Check sheet for the modelled part. Datum: model origin and axes. Units: mm. Face numbers are marked on the shaded views. A direction names the side the tool comes from. Give positions to 0.01 mm unless a question says otherwise; leave off trailing zeros. Order: outer loops, then holes, each group sorted by start corner. A loop starts at its lowest first (then second) coordinate and runs counter-clockwise, first axis right, second up.
```python
from build123d import *

# Parameters (mm, degrees)
SKETCH1_R                    = 27.125
BOSS_EXTRUDE1_DEPTH          = 6
CUT_EXTRUDE1_START           = 6
SKETCH2_R                    = 2.6
CUT_EXTRUDE1_DEPTH           = 45.826939745
CUT_EXTRUDE1_DRAFT           = 2
CUT_EXTRUDE1_PROFILE_2_DEPTH = 45.826939745
CUT_EXTRUDE1_PROFILE_2_DRAFT = 2
CUT_EXTRUDE1_PROFILE_3_DEPTH = 45.826939745
CUT_EXTRUDE1_PROFILE_3_DRAFT = 2
SKETCH2_R_2                  = 2.1
CUT_EXTRUDE1_PROFILE_4_DEPTH = 45.826939745
CUT_EXTRUDE1_PROFILE_4_DRAFT = 2
CUT_EXTRUDE1_PROFILE_5_DEPTH = 45.826939745
CUT_EXTRUDE1_PROFILE_5_DRAFT = 2
CUT_EXTRUDE1_PROFILE_6_DEPTH = 45.826939745
CUT_EXTRUDE1_PROFILE_6_DRAFT = 2
CUT_EXTRUDE1_PROFILE_7_DEPTH = 45.826939745
CUT_EXTRUDE1_PROFILE_7_DRAFT = 2
CUT_EXTRUDE1_PROFILE_8_DEPTH = 45.826939745
CUT_EXTRUDE1_PROFILE_8_DRAFT = 2
CUT_EXTRUDE1_PROFILE_9_DEPTH = 45.826939745
CUT_EXTRUDE1_PROFILE_9_DRAFT = 2


with BuildPart() as part:
    # Sketch1 → Boss-Extrude1 (new body)
    with BuildSketch(Plane(origin=(0, 0, 0), x_dir=(0, 1, 0), z_dir=(0, 0, 1))):
        with Locations(Location((0, 0, 0), (0, 0, 270))):
            Circle(SKETCH1_R)
    extrude(amount=BOSS_EXTRUDE1_DEPTH)


with BuildPart() as cut_extrude1_tool:
    # Sketch2 → Cut-Extrude1 (with draft: the straight prism first)
    with BuildSketch(Plane(origin=(0, 0, 6), x_dir=(1, 0, 0), z_dir=(0, 0, -1)).offset(CUT_EXTRUDE1_START)):
        with Locations((0, 16)):
            Circle(SKETCH2_R)
    extrude(amount=-CUT_EXTRUDE1_DEPTH)
    # Cut-Extrude1: the draft: its side faces are tilted about the plane it starts from
    cut_extrude1_sides = [cut_extrude1_tool.faces().sort_by_distance(p)[0] for p in [
        (-2.6, -16, 22.913469873),
    ]]
    draft(cut_extrude1_sides, Plane(origin=(0, 0, 6), x_dir=(1, 0, 0), z_dir=(0, 0, -1)).offset(CUT_EXTRUDE1_START), CUT_EXTRUDE1_DRAFT)


with BuildPart() as part_1:
    add(part.part)

    # Cut-Extrude1: cut by cut_extrude1_tool
    add(cut_extrude1_tool.part, mode=Mode.SUBTRACT)


with BuildPart() as cut_extrude1_profile_2_tool:
    # Sketch2 → Cut-Extrude1 profile 2 (with draft: the straight prism first)
    with BuildSketch(Plane(origin=(0, 0, 6), x_dir=(1, 0, 0), z_dir=(0, 0, -1)).offset(CUT_EXTRUDE1_START)):
        with Locations((13.856406461, -8)):
            Circle(SKETCH2_R)
    extrude(amount=-CUT_EXTRUDE1_PROFILE_2_DEPTH)
    # Cut-Extrude1 profile 2: the draft: its side faces are tilted about the plane it starts from
    cut_extrude1_profile_2_sides = [cut_extrude1_profile_2_tool.faces().sort_by_distance(p)[0] for p in [
        (11.256406461, 8, 22.913469873),
    ]]
    draft(cut_extrude1_profile_2_sides, Plane(origin=(0, 0, 6), x_dir=(1, 0, 0), z_dir=(0, 0, -1)).offset(CUT_EXTRUDE1_START), CUT_EXTRUDE1_PROFILE_2_DRAFT)


with BuildPart() as part_2:
    add(part_1.part)

    # Cut-Extrude1 profile 2: cut by cut_extrude1_profile_2_tool
    add(cut_extrude1_profile_2_tool.part, mode=Mode.SUBTRACT)


with BuildPart() as cut_extrude1_profile_3_tool:
    # Sketch2 → Cut-Extrude1 profile 3 (with draft: the straight prism first)
    with BuildSketch(Plane(origin=(0, 0, 6), x_dir=(1, 0, 0), z_dir=(0, 0, -1)).offset(CUT_EXTRUDE1_START)):
        with Locations((-13.856406461, -8)):
            Circle(SKETCH2_R)
    extrude(amount=-CUT_EXTRUDE1_PROFILE_3_DEPTH)
    # Cut-Extrude1 profile 3: the draft: its side faces are tilted about the plane it starts from
    cut_extrude1_profile_3_sides = [cut_extrude1_profile_3_tool.faces().sort_by_distance(p)[0] for p in [
        (-16.456406461, 8, 22.913469873),
    ]]
    draft(cut_extrude1_profile_3_sides, Plane(origin=(0, 0, 6), x_dir=(1, 0, 0), z_dir=(0, 0, -1)).offset(CUT_EXTRUDE1_START), CUT_EXTRUDE1_PROFILE_3_DRAFT)


with BuildPart() as part_3:
    add(part_2.part)

    # Cut-Extrude1 profile 3: cut by cut_extrude1_profile_3_tool
    add(cut_extrude1_profile_3_tool.part, mode=Mode.SUBTRACT)


with BuildPart() as cut_extrude1_profile_4_tool:
    # Sketch2 → Cut-Extrude1 profile 4 (with draft: the straight prism first)
    with BuildSketch(Plane(origin=(0, 0, 6), x_dir=(1, 0, 0), z_dir=(0, 0, -1)).offset(CUT_EXTRUDE1_START)):
        with Locations((-9, -15.588457268)):
            Circle(SKETCH2_R_2)
    extrude(amount=-CUT_EXTRUDE1_PROFILE_4_DEPTH)
    # Cut-Extrude1 profile 4: the draft: its side faces are tilted about the plane it starts from
    cut_extrude1_profile_4_sides = [cut_extrude1_profile_4_tool.faces().sort_by_distance(p)[0] for p in [
        (-11.1, 15.588457268, 22.913469873),
    ]]
    draft(cut_extrude1_profile_4_sides, Plane(origin=(0, 0, 6), x_dir=(1, 0, 0), z_dir=(0, 0, -1)).offset(CUT_EXTRUDE1_START), CUT_EXTRUDE1_PROFILE_4_DRAFT)


with BuildPart() as part_4:
    add(part_3.part)

    # Cut-Extrude1 profile 4: cut by cut_extrude1_profile_4_tool
    add(cut_extrude1_profile_4_tool.part, mode=Mode.SUBTRACT)


with BuildPart() as cut_extrude1_profile_5_tool:
    # Sketch2 → Cut-Extrude1 profile 5 (with draft: the straight prism first)
    with BuildSketch(Plane(origin=(0, 0, 6), x_dir=(1, 0, 0), z_dir=(0, 0, -1)).offset(CUT_EXTRUDE1_START)):
        with Locations((-18, 0)):
            Circle(SKETCH2_R_2)
    extrude(amount=-CUT_EXTRUDE1_PROFILE_5_DEPTH)
    # Cut-Extrude1 profile 5: the draft: its side faces are tilted about the plane it starts from
    cut_extrude1_profile_5_sides = [cut_extrude1_profile_5_tool.faces().sort_by_distance(p)[0] for p in [
        (-20.1, 0, 22.913469873),
    ]]
    draft(cut_extrude1_profile_5_sides, Plane(origin=(0, 0, 6), x_dir=(1, 0, 0), z_dir=(0, 0, -1)).offset(CUT_EXTRUDE1_START), CUT_EXTRUDE1_PROFILE_5_DRAFT)


with BuildPart() as part_5:
    add(part_4.part)

    # Cut-Extrude1 profile 5: cut by cut_extrude1_profile_5_tool
    add(cut_extrude1_profile_5_tool.part, mode=Mode.SUBTRACT)


with BuildPart() as cut_extrude1_profile_6_tool:
    # Sketch2 → Cut-Extrude1 profile 6 (with draft: the straight prism first)
    with BuildSketch(Plane(origin=(0, 0, 6), x_dir=(1, 0, 0), z_dir=(0, 0, -1)).offset(CUT_EXTRUDE1_START)):
        with Locations((-9, 15.588457268)):
            Circle(SKETCH2_R_2)
    extrude(amount=-CUT_EXTRUDE1_PROFILE_6_DEPTH)
    # Cut-Extrude1 profile 6: the draft: its side faces are tilted about the plane it starts from
    cut_extrude1_profile_6_sides = [cut_extrude1_profile_6_tool.faces().sort_by_distance(p)[0] for p in [
        (-11.1, -15.588457268, 22.913469873),
    ]]
    draft(cut_extrude1_profile_6_sides, Plane(origin=(0, 0, 6), x_dir=(1, 0, 0), z_dir=(0, 0, -1)).offset(CUT_EXTRUDE1_START), CUT_EXTRUDE1_PROFILE_6_DRAFT)


with BuildPart() as part_6:
    add(part_5.part)

    # Cut-Extrude1 profile 6: cut by cut_extrude1_profile_6_tool
    add(cut_extrude1_profile_6_tool.part, mode=Mode.SUBTRACT)


with BuildPart() as cut_extrude1_profile_7_tool:
    # Sketch2 → Cut-Extrude1 profile 7 (with draft: the straight prism first)
    with BuildSketch(Plane(origin=(0, 0, 6), x_dir=(1, 0, 0), z_dir=(0, 0, -1)).offset(CUT_EXTRUDE1_START)):
        with Locations((9, 15.588457268)):
            Circle(SKETCH2_R_2)
    extrude(amount=-CUT_EXTRUDE1_PROFILE_7_DEPTH)
    # Cut-Extrude1 profile 7: the draft: its side faces are tilted about the plane it starts from
    cut_extrude1_profile_7_sides = [cut_extrude1_profile_7_tool.faces().sort_by_distance(p)[0] for p in [
        (6.9, -15.588457268, 22.913469873),
    ]]
    draft(cut_extrude1_profile_7_sides, Plane(origin=(0, 0, 6), x_dir=(1, 0, 0), z_dir=(0, 0, -1)).offset(CUT_EXTRUDE1_START), CUT_EXTRUDE1_PROFILE_7_DRAFT)


with BuildPart() as part_7:
    add(part_6.part)

    # Cut-Extrude1 profile 7: cut by cut_extrude1_profile_7_tool
    add(cut_extrude1_profile_7_tool.part, mode=Mode.SUBTRACT)


with BuildPart() as cut_extrude1_profile_8_tool:
    # Sketch2 → Cut-Extrude1 profile 8 (with draft: the straight prism first)
    with BuildSketch(Plane(origin=(0, 0, 6), x_dir=(1, 0, 0), z_dir=(0, 0, -1)).offset(CUT_EXTRUDE1_START)):
        with Locations((18, 0)):
            Circle(SKETCH2_R_2)
    extrude(amount=-CUT_EXTRUDE1_PROFILE_8_DEPTH)
    # Cut-Extrude1 profile 8: the draft: its side faces are tilted about the plane it starts from
    cut_extrude1_profile_8_sides = [cut_extrude1_profile_8_tool.faces().sort_by_distance(p)[0] for p in [
        (15.9, 0, 22.913469873),
    ]]
    draft(cut_extrude1_profile_8_sides, Plane(origin=(0, 0, 6), x_dir=(1, 0, 0), z_dir=(0, 0, -1)).offset(CUT_EXTRUDE1_START), CUT_EXTRUDE1_PROFILE_8_DRAFT)


with BuildPart() as part_8:
    add(part_7.part)

    # Cut-Extrude1 profile 8: cut by cut_extrude1_profile_8_tool
    add(cut_extrude1_profile_8_tool.part, mode=Mode.SUBTRACT)


with BuildPart() as cut_extrude1_profile_9_tool:
    # Sketch2 → Cut-Extrude1 profile 9 (with draft: the straight prism first)
    with BuildSketch(Plane(origin=(0, 0, 6), x_dir=(1, 0, 0), z_dir=(0, 0, -1)).offset(CUT_EXTRUDE1_START)):
        with Locations((9, -15.588457268)):
            Circle(SKETCH2_R_2)
    extrude(amount=-CUT_EXTRUDE1_PROFILE_9_DEPTH)
    # Cut-Extrude1 profile 9: the draft: its side faces are tilted about the plane it starts from
    cut_extrude1_profile_9_sides = [cut_extrude1_profile_9_tool.faces().sort_by_distance(p)[0] for p in [
        (6.9, 15.588457268, 22.913469873),
    ]]
    draft(cut_extrude1_profile_9_sides, Plane(origin=(0, 0, 6), x_dir=(1, 0, 0), z_dir=(0, 0, -1)).offset(CUT_EXTRUDE1_START), CUT_EXTRUDE1_PROFILE_9_DRAFT)


with BuildPart() as part_9:
    add(part_8.part)

    # Cut-Extrude1 profile 9: cut by cut_extrude1_profile_9_tool
    add(cut_extrude1_profile_9_tool.part, mode=Mode.SUBTRACT)


solid = part_9.part
```
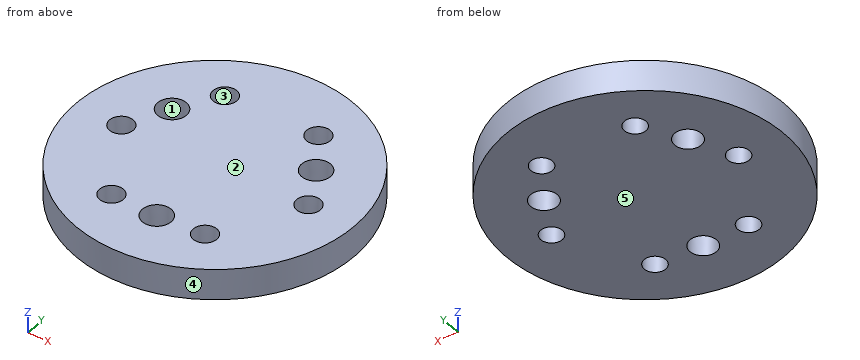
(1) Sectioned sample at B-B (y = 0). Enter the section's corners in (x, z) (3 decimals).
(2) Sectioned sample at A-A (x = 0). Enter the section's corners in (y, z) (3 decimals), plus the area to 3 significant figures.
(3) Thickness scan on L1, parallel to Y at x = -8.5, z = 3.6; L2, parallel to X at y = 16.5, z = 4.85; L3, parallel to X at y = -14, z = 5.5. Record the ranges inside material, lowest first.
(4) Go/stop test with flat-tipped pins: P1, Ø1, axis at x = -6.5, y = 7, coming from the -Z side; P2, Ø1, axis at x = -10, z = 4, coming from the +Y side; P3, Ø1, axis at x = -1, z = 5.5, coming from the +Y side; P4, Ø3, axis at y = -3, z = 2, coming from the +X side. Record where each tip stops, or that it passes through.
(5) Sectioned sample at D-D (x = 9). Enter the section's corners in (y, z), plus the area to 3 significant figures.
(6) Release check for a two-part mould opening along Y. For the marked faces 3, 4 and 5 record: released by +Y, released by -Y, zero draft, split by the parting line, or undercut.
(7) Tool access check on the marked faces 1 and 2. Record the directions out of +Z, -Z, +X, -X, +Y, -Y that give a thin tool (end or side, any length) a straight path to the whole face; none if there is none.
(8) Sectioned sample at C-C (z = 1.75). Count the separate pieces of the cut face and the enclosed holes in it, plus the area to 3 significant figures.
Values follow:
1. outline: (-27.125, 0) - (-20.1, 0) - (-20.31, 6) - (-27.125, 6) - close; (-15.9, 0) - (15.9, 0) - (15.69, 6) - (-15.69, 6) - close; (20.1, 0) - (27.125, 0) - (27.125, 6) - (20.31, 6) - close
2. outline: (-27.125, 0) - (-18.6, 0) - (-18.81, 6) - (-27.125, 6) - close; (-13.4, 0) - (27.125, 0) - (27.125, 6) - (-13.19, 6) - close
2. area: 293 mm2
3. L1: y = -25.76 to -17.76, -13.42 to 13.42, 17.76 to 25.76
3. L2: x = -21.53 to -11.08, -6.92 to 6.92, 11.08 to 21.53
3. L3: x = -23.23 to -10.65, -7.35 to -1.95, 1.95 to 7.35, 10.65 to 23.23
4. P1: stops at z = 0
4. P2: stops at y = 25.41
4. P3: stops at y = 27.12
4. P4: stops at x = 27.08
5. outline: (-25.59, 0) - (-17.69, 0) - (-17.9, 6) - (-25.59, 6) - close; (-13.49, 0) - (13.49, 0) - (13.28, 6) - (-13.28, 6) - close; (17.69, 0) - (25.59, 0) - (25.59, 6) - (17.9, 6) - close
5. area: 254 mm2
6. face 3: undercut
6. face 4: split by the parting line
6. face 5: zero draft
7. face 1: +Z
7. face 2: +Z, +X, -X, +Y, -Y
8. separate pieces: 1
8. enclosed holes: 9
8. area: 2,160 mm2
